Input: dimensioned drawing with shaded views. Units: mm. Origin: part minimum x, y, z. Coordinates: 2 decimals unless noted, no trailing zeros. Order: outer loops, then holes, each group sorted by start corner. A loop starts at its lowest first (then second) coordinate and runs counter-clockwise, first axis right, second up. Notation, with made-up numbers: (26.5, 17.25) -> (58.5, 17.25) arc R15 ccw to (58.5, 42.25) -> close; hole circle Ø9 at (-32.75, 17.5). An arc over 180 degrees is marked (long way). Answer in a Markdown table with one row per item. Add a question column.
1) Section query A-A on y = 22.5. Return the cut outline in (x, z).
2) Contact query for flat-ended pins moving along their axis: P1, Ø8, axis at y = 60.5, z = 14, coming from the -X side; P2, Ø1.5, axis at x = 22.5, z = 53.5, coming from the +Y side; P3, Ø3, axis at x = 18, y = 68, coming from the +Z side; P4, Ø3, axis at x = 5, y = 51, coming from the -Z side. Output: stop coordinate, or through.
3) Section query C-C on x = 4. Return the cut outline in (y, z), then the cut area to 3 significant figures.
4) Section query B-B on z = 20. Return the cut outline in (x, y).
5) Ray query, line 1 (Y direction, x = 7.75, z = 56); line 2 (Y direction, x = 4.5, z = 28.5); line 3 (Z direction, x = 18.75, y = 30). Return the intervals inside material, ascending. Write a range as from..to.
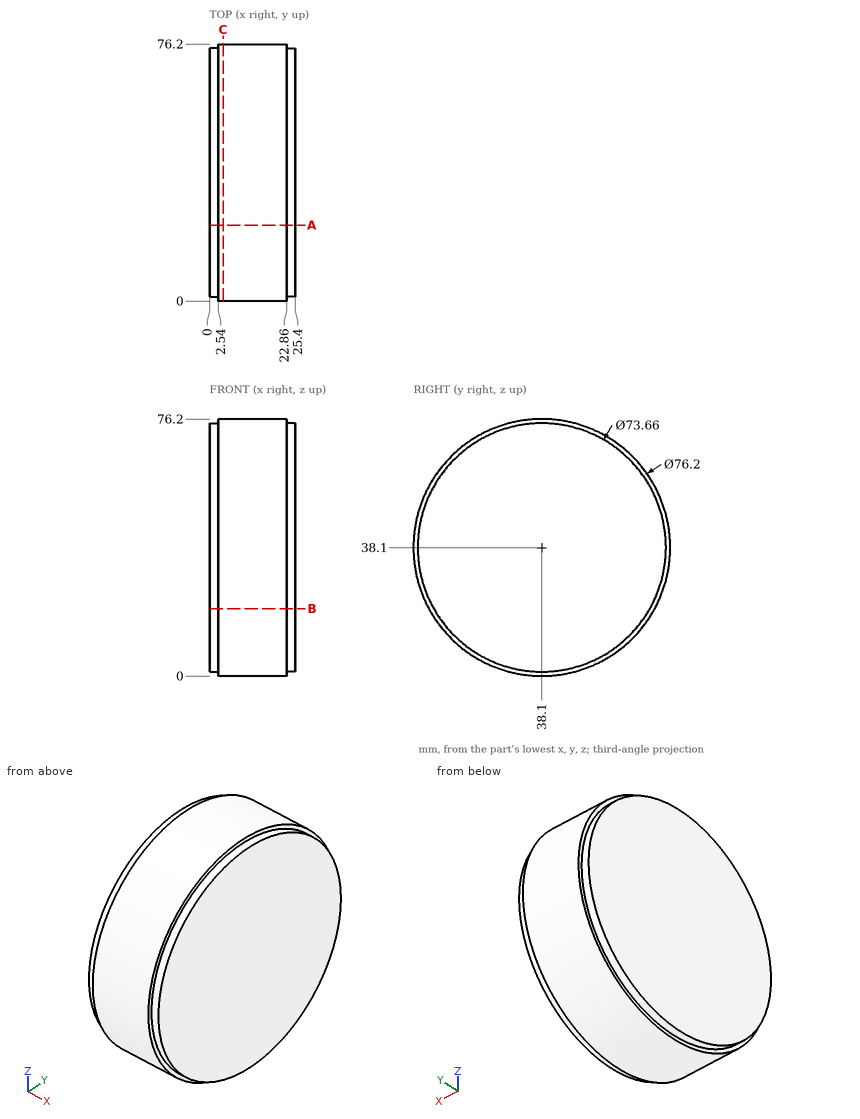
Result:
| question | item | result |
|---|---|---|
| 1 | outline | (0, 4.74) -> (2.54, 4.74) -> (2.54, 3.34) -> (22.86, 3.34) -> (22.86, 4.74) -> (25.4, 4.74) -> (25.4, 71.46) -> (22.86, 71.46) -> (22.86, 72.86) -> (2.54, 72.86) -> (2.54, 71.46) -> (0, 71.46) -> close |
| 2 | P1 | x = 0 |
| 2 | P2 | y = 73.27 |
| 2 | P3 | z = 63.5 |
| 2 | P4 | z = 1.75 |
| 3 | outline | circle Ø76.2 at (38.1, 38.1) |
| 3 | area | 4,560 mm2 |
| 4 | outline | (0, 6.02) -> (2.54, 6.02) -> (2.54, 4.57) -> (22.86, 4.57) -> (22.86, 6.02) -> (25.4, 6.02) -> (25.4, 70.18) -> (22.86, 70.18) -> (22.86, 71.63) -> (2.54, 71.63) -> (2.54, 70.18) -> (0, 70.18) -> close |
| 5 | line 1 | 4.47..71.73 |
| 5 | line 2 | 1.23..74.97 |
| 5 | line 3 | 0.87..75.33 |
